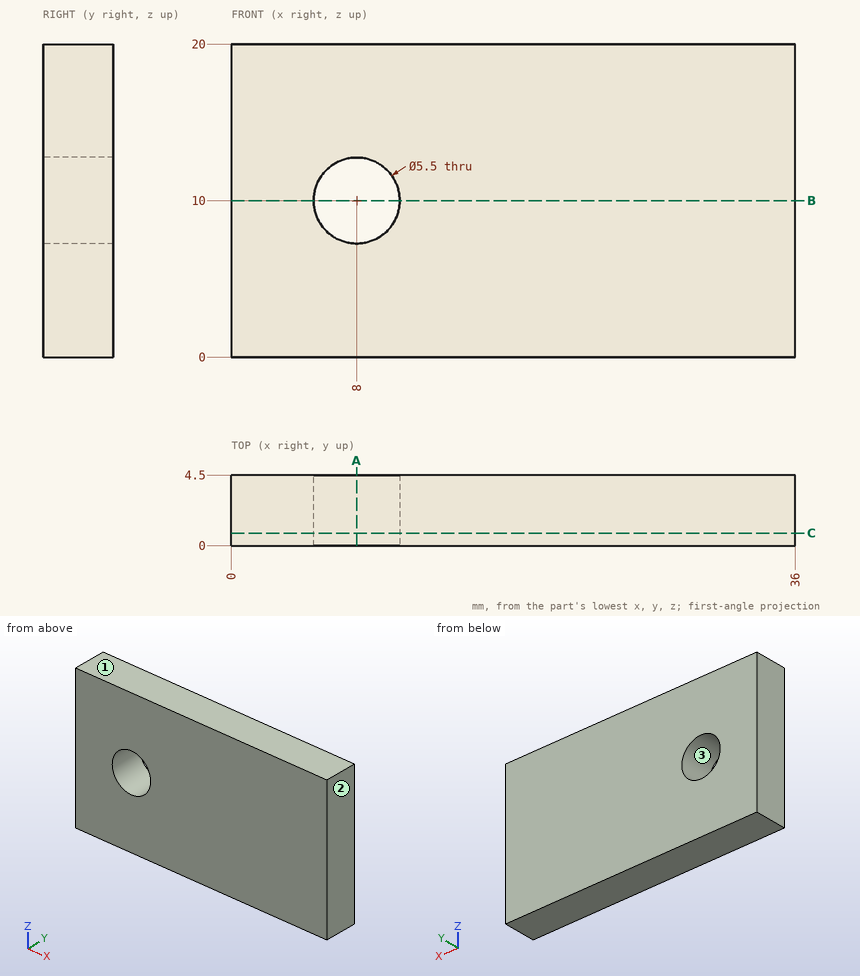
The figure shows three views and two pictorial views of one solid part (mm, origin at its lowest corner). Answer the questions. Coordinates: 2 decimals unless noted, no trailing zeros. Loops run counter-clockwise (first coordinate to the right, second up) from the corner with the lowest first, then second, coordinate; pieces in that order, holes last. Notation, with made-up numbers: (-4.75, 3) -> (32.25, 3) arc R14 ccw to (32.25, 24) -> close; hole circle Ø2 at (83.25, 87.5). An arc over 180 degrees is marked (long way). Return JSON: item names as keys, results as strings. Group by question number.
(1) Find the intervals of material crossed by probe 1 along Z at (x, y) = (8, 3.4); probe 2 along X at (y, z) = (2.3, 10); probe 3 along X at (y, z) = (1.85, 12.5), in increasing order. Write a range as from..to.
(2) A cutting plane is placed at C-C on y = 0.8. Write down the section's boundary in (x, z).
(3) Determine the mould class of the marked faces 1, 2 and 3 for opening direction Z: released by +Z, released by -Z, zero draft, split by the parting line, or undercut.
(4) A cutting plane is placed at A-A on x = 8. Write down the section's boundary in (y, z).
(5) A cutting plane is placed at B-B on z = 10. Write down the section's boundary in (x, y), and give its area (3 significant figures).
The answers:
{
 "1": {"probe 1": "z = 0..7.25, 12.75..20", "probe 2": "x = 0..5.25, 10.75..36", "probe 3": "x = 0..6.85, 9.15..36"},
 "2": {"outline": "(0, 0) -> (36, 0) -> (36, 20) -> (0, 20) -> close; hole circle Ø5.5 at (8, 10)"},
 "3": {"face 1": "released by +Z", "face 2": "zero draft", "face 3": "undercut"},
 "4": {"outline": "(0, 0) -> (4.5, 0) -> (4.5, 7.25) -> (0, 7.25) -> close; (0, 12.75) -> (4.5, 12.75) -> (4.5, 20) -> (0, 20) -> close"},
 "5": {"outline": "(0, 0) -> (5.25, 0) -> (5.25, 4.5) -> (0, 4.5) -> close; (10.75, 0) -> (36, 0) -> (36, 4.5) -> (10.75, 4.5) -> close", "area": "137 mm^2"}
}
